Input: part model. Units: mm. Frame: model coordinates. A direction names the side the tool comes from. Coordinates: 2 decimals unless noted, no trailing zeros. Order: outer loops, then holes, each group sorted by start corner. A loop starts at its lowest first (then second) coordinate and runs counter-clockwise, first axis right, second up. Notation, with made-up numbers: (10, 44.25) - (17, 44.25) arc R20 cw to (17, 58.25) - close; hole circle Ø5 at (-7.75, -9.75). An arc over 180 degrees is marked (long way). Use a Markdown table: item, result. Add a question column.
from build123d import *

# Parameters (mm, degrees)
BOSS_EXTRUDE1_DEPTH = 10
SKETCH2_R           = 3
BOSS_EXTRUDE2_DEPTH = 2.5
SKETCH4_W           = 2.5
SKETCH4_H           = 32
BOSS_EXTRUDE3_DEPTH = 60
SKETCH5_R           = 5
CUT_EXTRUDE1_DEPTH  = 10


with BuildPart() as part:
    # Sketch1 → Boss-Extrude1 (new body)
    with BuildSketch(Plane(origin=(0, 0, 0), x_dir=(1, 0, 0), z_dir=(0, 1, 0))):
        with BuildLine():
            Line((-24.017268371, 4.839506173), (-15.684746691, 3.160493827))
            ThreePointArc((-15.684746691, 3.160493827), (0, 16), (15.684746691, 3.160493827))
            Line((15.684746691, 3.160493827), (24.017268371, 4.839506173))
            ThreePointArc((24.017268371, 4.839506173), (0, 24.5), (-24.017268371, 4.839506173))
        make_face()
    extrude(amount=BOSS_EXTRUDE1_DEPTH)

    # Sketch2 → Boss-Extrude2 (add)
    with BuildSketch(Plane.XZ):
        with BuildLine():
            Line((37.5, -16), (37.5, 16))
            Line((37.5, 16), (21.748563171, 16))
            ThreePointArc((21.748563171, 16), (12.186057607, 24.093567606), (0, 27))
            ThreePointArc((0, 27), (-27, 0), (0, -27))
            ThreePointArc((0, -27), (12.186057607, -24.093567606), (21.748563171, -16))
            Line((21.748563171, -16), (37.5, -16))
        make_face()
        with Locations(Location((0, 0, 0), (0, 0, 270))):
            Circle(SKETCH2_R, mode=Mode.SUBTRACT)
    extrude(amount=BOSS_EXTRUDE2_DEPTH)

    # Sketch4 → Boss-Extrude3 (add)
    with BuildSketch(Plane(origin=(0, 0, 0), x_dir=(1, 0, 0), z_dir=(0, 1, 0))):
        with Locations((36.25, 0)):
            Rectangle(SKETCH4_W, SKETCH4_H)
    extrude(amount=BOSS_EXTRUDE3_DEPTH)

    # Sketch5 → Cut-Extrude1 (cut)
    with BuildSketch(Plane(origin=(37.5, 0, 0), x_dir=(0, 0, -1), z_dir=(1, 0, 0))):
        with Locations((0, 28.75)):
            Circle(SKETCH5_R)
    extrude(amount=-CUT_EXTRUDE1_DEPTH, mode=Mode.SUBTRACT)


solid = part.part
1) Material intervals for L1, parallel to X at y = -1.35, z = 0; L2, parallel to X at y = 6.5, z = -7; L3, parallel to X at y = 12, z = 4.5, sorted ascending.
2) Contact query for flat-ended pins moving along their axis: P1, Ø5, axis at x = -15, z = 18, coming from the +Y side; P2, Ø5, axis at x = 0, z = 0, coming from the +Y side; P3, Ø17.5, axis at x = 28, y = 21, coming from the -Z side; P4, Ø9.5, axis at y = 35, z = -4, coming from the -X side. Output: stop coordinate, or through.
3) Cut plane D-D (y = 15.5). Return the cut outline in (x, z), and give its area (3 significant figures).
4) Pull-direction query (Z, two-part tool) for faces 6 (the cylindrical face through (36.27, 23.87, 1.08)), 7 (the flat face through (19.793, 4.93, -3.988)), 8 (the flat face through (-0.3, 10, -16.4)); classes: pulls with the +Z half, pulls with the -Z half, needs draft (parallel to the pull), parting line crosses it, or undercut.
5) Reachability of faces 1 (the flat face through (36, 24, 16)), 2 (the cylindrical face through (0, 5, -16)), 3 (the flat face through (-19.91, 4.93, -4.01)), 4 (the flat face through (36, 24, -16)), 5 (the cylindrical face through (0.471, 4.93, -24.495)) from +Z, -Z, +X, -X, +Y, -Y: full face, straight path, thin tool, end or side. Return the list, or none.
6) Cut plane A-A (y = 28.75). Return the cut outline in (x, z).
7) Cut plane C-C (x = 31). Return the cut outline in (y, z), and give its area (3 significant figures).
8) Cut plane B-B (z = 0). Return the cut outline in (x, y).
Computed:
| question | item | result |
|---|---|---|
| 1 | L1 | x = -27 to -3, 3 to 37.5 |
| 1 | L2 | x = -23.48 to -14.39, 14.39 to 23.48, 35 to 37.5 |
| 1 | L3 | x = 35 to 37.5 |
| 2 | P1 | stops at y = 0 |
| 2 | P2 | passes through |
| 2 | P3 | stops at z = -16 |
| 2 | P4 | stops at x = 35 |
| 3 | outline | (35, -16) - (37.5, -16) - (37.5, 16) - (35, 16) - close |
| 3 | area | 80.0 mm2 |
| 4 | face 6 | undercut |
| 4 | face 7 | pulls with the +Z half |
| 4 | face 8 | needs draft |
| 5 | face 1 | +Z, +X, +Y, -Y |
| 5 | face 2 | +Z, +Y |
| 5 | face 3 | +Z, -X, +Y |
| 5 | face 4 | -Z, +X, +Y, -Y |
| 5 | face 5 | -Z, +Y |
| 6 | outline | (35, -16) - (37.5, -16) - (37.5, -5) - (35, -5) - close; (35, 5) - (37.5, 5) - (37.5, 16) - (35, 16) - close |
| 7 | outline | (-2.5, -16) - (0, -16) - (0, 16) - (-2.5, 16) - close |
| 7 | area | 80.0 mm2 |
| 8 | outline | (-27, -2.5) - (-3, -2.5) - (-3, 0) - (-27, 0) - close; (3, -2.5) - (37.5, -2.5) - (37.5, 23.75) - (35, 23.75) - (35, 0) - (3, 0) - close; (35, 33.75) - (37.5, 33.75) - (37.5, 60) - (35, 60) - close |
